Autodesk Inventor part; units mm, degrees
ref_plane "YZ Plane" through (0, 0, 0) normal (1, 0, 0) x (0, 1, 0)
ref_plane "XZ Plane" through (0, 0, 0) normal (0, 1, 0) x (-1, 0, 0)
ref_plane "XY Plane" through (0, 0, 0) normal (0, 0, 1) x (1, 0, 0)
sketch "Sketch1" plane through (0, 0, 0) normal (0, 1, 0) x (-1, 0, 0)
  line L0 (0, 0) -> (40, 0)
  line L1 (40, 0) -> (40, -50)
  line L2 (40, -50) -> (0, -50)
  line L3 (0, -50) -> (0, 0)
  circle A0 centre (20, -10) radius 2.5
  circle A1 centre (20, -40) radius 2.5
  dimension "d0" = 40
  dimension "d1" = 50
  dimension "d2" = 5
  dimension "d3" = 5
  dimension "d4" = 10
  dimension "d5" = 10
  dimension "d6" = 20
extrude "Extrusion1" add sketch "Sketch1" along normal blind 5
sketch "Sketch2" plane through (0, 5, 0) normal (0, 1, 0) x (1, 0, 0)
  line L0 (-40, 50) -> (-40, 0)
  line L1 (0, 0) -> (0, 50)
  line L2 (-40, 22.5) -> (0, 22.5)
  line L3 (0, 22.5) -> (0, 27.5)
  line L4 (0, 27.5) -> (-40, 27.5)
  line L5 (-40, 27.5) -> (-40, 22.5)
  line L6 (-40, 0) -> (0, 0)
  line L7 (0, 50) -> (-40, 50)
  line L8 (-40, 50) -> (-35, 50)
  line L9 (-35, 50) -> (-35, 0)
  line L10 (-35, 0) -> (-40, 0)
  line L11 (-40, 0) -> (-40, 50)
  line L12 (-5, 0) -> (0, 0)
  line L13 (0, 0) -> (0, 50)
  line L14 (0, 50) -> (-5, 50)
  line L15 (-5, 50) -> (-5, 0)
  point P0 (0, 22.5)
  point P1 (-5, 22.5)
  point P2 (-5, 27.5)
  point P3 (-35, 22.5)
  point P4 (-35, 27.5)
  dimension "d9" = 5
  dimension "d10" = 22.5
  dimension "d13" = 5
  dimension "d14" = 5
extrude "Extrusion2" add sketch "Sketch2" along normal blind 20 contours L7 L9 L4 L0 | L4 L9 L2 L0 | L2 L9 L6 L0 | L4 L15 L2 L9 | L7 L1 L4 L15 | L4 L1 L2 L15 | L2 L1 L6 L15
fillet "Fillet1" radius 22.25 4 edges at (-37.5, 25, 0) (-37.5, 25, -50) (-2.5, 25, -50) (-2.5, 25, 0)
properties part number "LightSensor01"
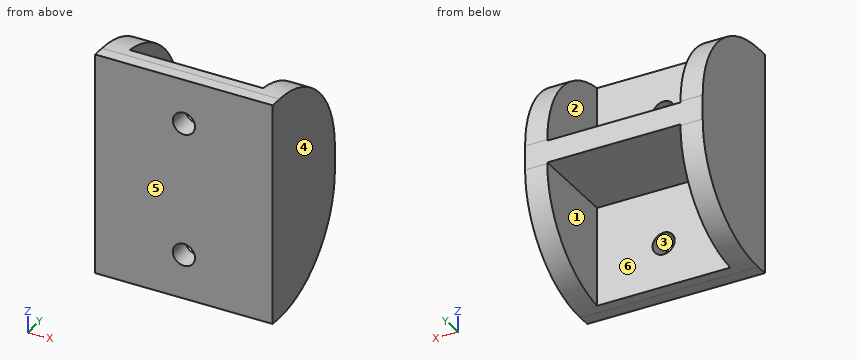
Here's how the part is built. I have some questions about the finished solid (model axes, mm). Face numbers are marked on the shaded views. A direction names the side the tool comes from. Give positions to 0.01 mm unless a question says otherwise; leave off trailing zeros. Write each loop counter-clockwise with the first axis right and the second up, starting at its lowest first coordinate (ties: lowest second). Pieces come first, ordered by that corner, then holes. Notation, with made-up numbers: (29.5, 43.25) -> (40.5, 43.25) arc R32 cw to (40.5, 71.25) -> close; hole circle Ø3 at (-25, -19.5). An arc over 180 degrees is marked (long way). Use one line per item in the form item = value. Start each with the question number.
1. Imagine slicing it at C-C on x = -11. List the corners of the cut face in (y, z) for me, plus the area to 3 significant figures.
2. Thinking about a two-plate mould opening in X: for the marked faces 4, 5 and 6, which applies, +X half, -X half, draft (parallel to the pull), parting line (faces both ways), or undercut?
3. Will these pins go through, and if not, where does the flat tip stop? pin 1 Ø10 at (x, z) = (-11, -44) entering from +Y; pin 2 Ø10 at (x, y) = (-24, 15.5) entering from -Z; pin 3 Ø6 at (x, y) = (-27.5, 7) entering from -Z; pin 4 Ø4.5 at (x, z) = (-20, -10) entering from +Y.
4. On a 3-axis mill with a long thin cutter (end or side, diameter ignored), from which of +Z, -Z, +X, -X, +Y, -Y can I reach the whole of each face in a straight line? I mean the marked faces 1, 2 and 3. Say none if no direction works.
5. Imagine slicing it at D-D on y = 17.25. List the corners of the cut face in (x, z) for me, plus the area to 3 significant figures.
6. Imagine slicing it at B-B on z = -40. List the corners of the cut face in (x, y) for me, plus the area to 3 significant figures.
7. Imagine slicing it at A-A on x = -20. List the corners of the cut face in (y, z) for me.
8. If I drill on L1, parallel to Z at x = -20, y = 1.1; L2, parallel to X at y = 17, z = -21; L3, parallel to Z at x = -22.5, y = 13, over which ranges is the centre line in solid material (lowest first)?
Entries:
q1.outline = (0, -50) -> (2.75, -50) arc R22.25 ccw to (5, -49.89) -> (5, -27.5) -> (25, -27.5) -> (25, -22.5) -> (5, -22.5) -> (5, -0.11) arc R22.25 ccw to (2.75, 0) -> (0, 0) -> close
q1.area = 350 mm²
q2.face_4 = +X half
q2.face_5 = draft
q2.face_6 = undercut
q3.pin_1 = 5
q3.pin_2 = -27.5
q3.pin_3 = -49.96
q3.pin_4 = through
q4.face_1 = -Z, +Y
q4.face_2 = +Z, +Y
q4.face_3 = +Y, -Y
q5.outline = (-40, -44.63) -> (-35, -44.63) -> (-35, -27.5) -> (-5, -27.5) -> (-5, -44.63) -> (0, -44.63) -> (0, -5.37) -> (-5, -5.37) -> (-5, -22.5) -> (-35, -22.5) -> (-35, -5.37) -> (-40, -5.37) -> close
q5.area = 543 mm²
q6.outline = (-40, 0) -> (-22.5, 0) -> (-22.5, 5) -> (-35, 5) -> (-35, 21.32) -> (-40, 21.32) -> close; (-17.5, 0) -> (0, 0) -> (0, 21.32) -> (-5, 21.32) -> (-5, 5) -> (-17.5, 5) -> close
q6.area = 338 mm²
q7.outline = (0, -50) -> (2.75, -50) arc R22.25 ccw to (5, -49.89) -> (5, -42.5) -> (0, -42.5) -> close; (0, -37.5) -> (5, -37.5) -> (5, -27.5) -> (25, -27.5) -> (25, -22.5) -> (5, -22.5) -> (5, -12.5) -> (0, -12.5) -> close; (0, -7.5) -> (5, -7.5) -> (5, -0.11) arc R22.25 ccw to (2.75, 0) -> (0, 0) -> close
q8.L1 = -50 to -42.5, -37.5 to -12.5, -7.5 to 0
q8.L2 = -40 to -35, -5 to 0
q8.L3 = -27.5 to -22.5
